The listing builds one solid part. Answer for the finished solid, in the listing's coordinates (mm). A direction names the side the tool comes from. Coordinates: 2 decimals unless noted, no trailing zeros. Loops run counter-clockwise (first coordinate to the right, second up) from the corner with the lowest first, then second, coordinate; pieces in that order, holes last. Notation, with made-up numbers: (72.5, -21.5) - (78.5, -21.5) arc R29 cw to (78.5, 9.5) - close; hole circle Ø2 at (48.5, 52). An arc over 180 degrees is marked (long way). Put each result on its own line as item: value.
```python
from build123d import *

# Parameters (mm, degrees)
CROQUIS1_W              = 16.3
CROQUIS1_H              = 3
CROQUIS1_W_2            = 3
CROQUIS1_H_2            = 12.3
SALIENTE_EXTRUIR1_DEPTH = 3
CORTAR_EXTRUIR1_REACH   = 5
CROQUIS2_R              = 1.4
CORTAR_EXTRUIR2_REACH   = 5
CROQUIS3_R              = 1.4


with BuildPart() as part:
    # Croquis1 → Saliente-Extruir1 (new body)
    with BuildSketch(Plane(origin=(0, 0, 0), x_dir=(1, 0, 0), z_dir=(0, 1, 0))):
        with BuildLine():
            Line((-54, 45.5), (54, 45.5))
            ThreePointArc((54, 45.5), (55.414213562, 44.914213562), (56, 43.5))
            Line((56, 43.5), (56, -43.5))
            ThreePointArc((56, -43.5), (55.414213562, -44.914213562), (54, -45.5))
            Line((54, -45.5), (-54, -45.5))
            ThreePointArc((-54, -45.5), (-55.414213562, -44.914213562), (-56, -43.5))
            Line((-56, -43.5), (-56, 43.5))
            ThreePointArc((-56, 43.5), (-55.414213562, 44.914213562), (-54, 45.5))
        make_face()
        with Locations((-27.15, 41.5)):
            Rectangle(CROQUIS1_W, CROQUIS1_H, mode=Mode.SUBTRACT)
        with Locations((27.15, 41.5)):
            Rectangle(CROQUIS1_W, CROQUIS1_H, mode=Mode.SUBTRACT)
        with Locations((-27.15, -41.5)):
            Rectangle(CROQUIS1_W, CROQUIS1_H, mode=Mode.SUBTRACT)
        with Locations((27.15, -41.5)):
            Rectangle(CROQUIS1_W, CROQUIS1_H, mode=Mode.SUBTRACT)
        with Locations((51.5, 25.65)):
            Rectangle(CROQUIS1_W_2, CROQUIS1_H_2, mode=Mode.SUBTRACT)
        with Locations((51.5, -25.65)):
            Rectangle(CROQUIS1_W_2, CROQUIS1_H_2, mode=Mode.SUBTRACT)
        with Locations((-51.5, 25.65)):
            Rectangle(CROQUIS1_W_2, CROQUIS1_H_2, mode=Mode.SUBTRACT)
        with Locations((-51.5, -25.65)):
            Rectangle(CROQUIS1_W_2, CROQUIS1_H_2, mode=Mode.SUBTRACT)
    extrude(amount=SALIENTE_EXTRUIR1_DEPTH)

    # Croquis2 → Cortar-Extruir1 (cut, up to next)
    with BuildSketch(Plane.XZ, mode=Mode.PRIVATE) as cortar_extruir1_sk1:
        with Locations((53, -42)):
            Circle(CROQUIS2_R)
    cortar_extruir1_tool1 = extrude(cortar_extruir1_sk1.sketch, amount=-CORTAR_EXTRUIR1_REACH, mode=Mode.PRIVATE) & part.part
    add(cortar_extruir1_tool1.solids().sort_by_distance((53, 0, -42))[0], mode=Mode.SUBTRACT)
    # Croquis2 → Cortar-Extruir1 (cut, up to next)
    with BuildSketch(Plane.XZ, mode=Mode.PRIVATE) as cortar_extruir1_sk2:
        with Locations((-52.5, -42)):
            Circle(CROQUIS2_R)
    cortar_extruir1_tool2 = extrude(cortar_extruir1_sk2.sketch, amount=-CORTAR_EXTRUIR1_REACH, mode=Mode.PRIVATE) & part.part
    add(cortar_extruir1_tool2.solids().sort_by_distance((-52.5, 0, -42))[0], mode=Mode.SUBTRACT)
    # Croquis2 → Cortar-Extruir1 (cut, up to next)
    with BuildSketch(Plane.XZ, mode=Mode.PRIVATE) as cortar_extruir1_sk3:
        with Locations((-52.5, 42)):
            Circle(CROQUIS2_R)
    cortar_extruir1_tool3 = extrude(cortar_extruir1_sk3.sketch, amount=-CORTAR_EXTRUIR1_REACH, mode=Mode.PRIVATE) & part.part
    add(cortar_extruir1_tool3.solids().sort_by_distance((-52.5, 0, 42))[0], mode=Mode.SUBTRACT)
    # Croquis2 → Cortar-Extruir1 (cut, up to next)
    with BuildSketch(Plane.XZ, mode=Mode.PRIVATE) as cortar_extruir1_sk4:
        with Locations((53, 42)):
            Circle(CROQUIS2_R)
    cortar_extruir1_tool4 = extrude(cortar_extruir1_sk4.sketch, amount=-CORTAR_EXTRUIR1_REACH, mode=Mode.PRIVATE) & part.part
    add(cortar_extruir1_tool4.solids().sort_by_distance((53, 0, 42))[0], mode=Mode.SUBTRACT)

    # Croquis3 → Cortar-Extruir2 (cut, up to next)
    with BuildSketch(Plane(origin=(0, 0, 0), x_dir=(1, 0, 0), z_dir=(0, 1, 0)), mode=Mode.PRIVATE) as cortar_extruir2_sk1:
        with Locations((40, -22.5)):
            Circle(CROQUIS3_R)
    cortar_extruir2_tool1 = extrude(cortar_extruir2_sk1.sketch, amount=CORTAR_EXTRUIR2_REACH, mode=Mode.PRIVATE) & part.part
    add(cortar_extruir2_tool1.solids().sort_by_distance((40, 0, 22.5))[0], mode=Mode.SUBTRACT)
    # Croquis3 → Cortar-Extruir2 (cut, up to next)
    with BuildSketch(Plane(origin=(0, 0, 0), x_dir=(1, 0, 0), z_dir=(0, 1, 0)), mode=Mode.PRIVATE) as cortar_extruir2_sk2:
        with Locations((40, 35.5)):
            Circle(CROQUIS3_R)
    cortar_extruir2_tool2 = extrude(cortar_extruir2_sk2.sketch, amount=CORTAR_EXTRUIR2_REACH, mode=Mode.PRIVATE) & part.part
    add(cortar_extruir2_tool2.solids().sort_by_distance((40, 0, -35.5))[0], mode=Mode.SUBTRACT)
    # Croquis3 → Cortar-Extruir2 (cut, up to next)
    with BuildSketch(Plane(origin=(0, 0, 0), x_dir=(1, 0, 0), z_dir=(0, 1, 0)), mode=Mode.PRIVATE) as cortar_extruir2_sk3:
        with Locations((-46, 35.5)):
            Circle(CROQUIS3_R)
    cortar_extruir2_tool3 = extrude(cortar_extruir2_sk3.sketch, amount=CORTAR_EXTRUIR2_REACH, mode=Mode.PRIVATE) & part.part
    add(cortar_extruir2_tool3.solids().sort_by_distance((-46, 0, -35.5))[0], mode=Mode.SUBTRACT)
    # Croquis3 → Cortar-Extruir2 (cut, up to next)
    with BuildSketch(Plane(origin=(0, 0, 0), x_dir=(1, 0, 0), z_dir=(0, 1, 0)), mode=Mode.PRIVATE) as cortar_extruir2_sk4:
        with Locations((-46, -22.5)):
            Circle(CROQUIS3_R)
    cortar_extruir2_tool4 = extrude(cortar_extruir2_sk4.sketch, amount=CORTAR_EXTRUIR2_REACH, mode=Mode.PRIVATE) & part.part
    add(cortar_extruir2_tool4.solids().sort_by_distance((-46, 0, 22.5))[0], mode=Mode.SUBTRACT)


solid = part.part
```
1) For faces 1 (the face through (27, 1, 40)), 2 (the face through (1, 3, -1)), determine the directions among +Z, -Z, +X, -X, +Y, -Y from which every point of the face is accessible in a straight line to the end or side of a thin tool.
Found:
face 1: +Y, -Y
face 2: +Z, -Z, +X, -X, +Y
2) For a pull along X with two mould halves and no side action, classify faces 3 (the face through (-19, 1, 42)), 4 (the face through (-1, 1, -45.5)), 5 (the face through (-56, 1, 1)) as pulls with the +X half, pulls with the -X half, needs draft (parallel to the pull), parting line crosses it, or undercut.
Found:
face 3: undercut
face 4: needs draft
face 5: pulls with the -X half
3) The part is cut by section A-A (z = 22.5). Give the vertices of the cut face in (x, y), and give its area (3 significant figures).
Found:
outline: (-56, 0) - (-53, 0) - (-53, 3) - (-56, 3) - close; (-50, 0) - (-47.4, 0) - (-47.4, 3) - (-50, 3) - close; (-44.6, 0) - (38.6, 0) - (38.6, 3) - (-44.6, 3) - close; (41.4, 0) - (50, 0) - (50, 3) - (41.4, 3) - close; (53, 0) - (56, 0) - (56, 3) - (53, 3) - close
area: 301 mm^2
4) The part is cut by section D-D (y = 0.6). State how many separate pieces and enclosed holes the cut face has, and give its area (3 significant figures).
Found:
separate pieces: 1
enclosed holes: 16
area: 9,800 mm^2
5) The part is cut by section C-C (x = -30). Give the vertices of the cut face in (y, z), and give its area (3 significant figures).
Found:
outline: (0, -45.5) - (3, -45.5) - (3, -43) - (0, -43) - close; (0, -40) - (3, -40) - (3, 40) - (0, 40) - close; (0, 43) - (3, 43) - (3, 45.5) - (0, 45.5) - close
area: 255 mm^2
6) Straight lines are drawn through the part: L1, parallel to Z at x = -52.5, y = 1.55; L2, parallel to Z at x = 50.5, y = 1.3; L3, parallel to X at y = 1.55, z = -35.5. For each, find the intervals that lie inside material, in ascending order. Write a range as [from, to].
Found:
L1: z = [-45.5, -43.4], [-40.6, -31.8], [-19.5, 19.5], [31.8, 40.6], [43.4, 45.5]
L2: z = [-45.5, -31.8], [-19.5, 19.5], [31.8, 45.5]
L3: x = [-56, -47.4], [-44.6, 38.6], [41.4, 56]
7) The part is cut by section B-B (z = -30.5). Give the vertices of the cut face in (x, y), and give its area (3 significant figures).
Found:
outline: (-56, 0) - (-53, 0) - (-53, 3) - (-56, 3) - close; (-50, 0) - (50, 0) - (50, 3) - (-50, 3) - close; (53, 0) - (56, 0) - (56, 3) - (53, 3) - close
area: 318 mm^2
